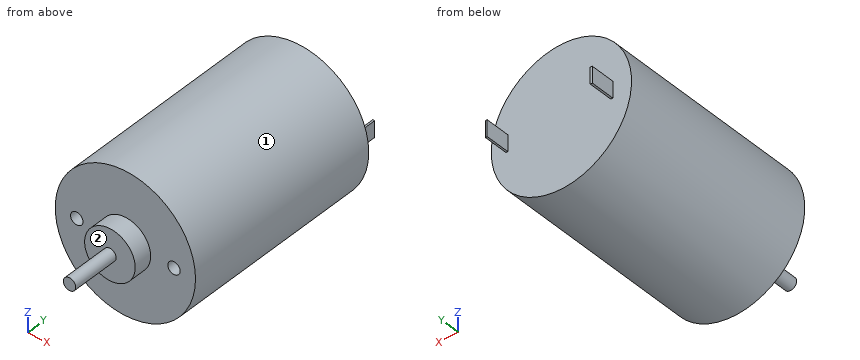
Autodesk Inventor part; units mm, degrees
ref_plane "YZ Plane" through (0, 0, 0) normal (1, 0, 0) x (0, 1, 0)
ref_plane "XZ Plane" through (0, 0, 0) normal (0, 1, 0) x (-1, 0, 0)
ref_plane "XY Plane" through (0, 0, 0) normal (0, 0, 1) x (1, 0, 0)
sketch "Sketch1" plane through (0, 0, 0) normal (0, 0, 1) x (1, 0, 0)
  line L0 (0, 0) -> (1.6, 0)
  line L1 (1.6, 0) -> (1.6, 12.446)
  line L2 (0, 17.2085) -> (18.034, 17.2085)
  line L3 (0, 12.446) -> (6.5, 12.446)
  line L4 (6.5, 12.446) -> (6.5, 17.2085)
  line L5 (18.034, 17.2085) -> (18.034, 70.5485)
  line L6 (18.034, 70.5485) -> (0, 70.5485)
  line L7 (0, 70.5485) -> (0, 0)
  dimension "d0" = 1.6
  dimension "d1" = 12.446
  dimension "d2" = 18.034
  dimension "d3" = 6.5
  dimension "d4" = 4.7625
  dimension "d5" = 53.34
revolve "Revolution1" add sketch "Sketch1" angle 360 about axis through (0, 70.5485, 0) along (0, -1, 0)
sketch "Sketch2" plane through (0, 17.2085, 0) normal (0, -1, 0) x (1, 0, 0)
  circle A0 centre (0, 0) radius 12.5
  circle A1 centre (-12.5, 0) radius 1.6
  circle A2 centre (12.5, 0) radius 1.6
  point P0 (0, 0)
  dimension "d7" = 25
  dimension "d8" = 3.2
  dimension "d9" = 3.2
extrude "Extrusion1" cut sketch "Sketch2" against normal blind 6.35 contours A0 A2 | A0 A2 | A1 A0 | A0 A1
sketch "Sketch3" plane through (0, 70.5485, 0) normal (0, 1, 0) x (1, 0, 0)
  line L0 (14.2427, 1.9025) -> (13.7699, 1.9025)
  line L1 (13.7699, 1.9025) -> (13.7699, -2.2939)
  line L2 (13.7699, -2.2939) -> (14.2427, -2.2939)
  line L3 (14.2427, -2.2939) -> (14.2427, 1.9025)
  line L4 (-12.709, 1.9025) -> (-13.2409, 1.9025)
  line L5 (-13.2409, 1.9025) -> (-13.2409, -2.2939)
  line L6 (-13.2409, -2.2939) -> (-12.709, -2.2939)
  line L7 (-12.709, -2.2939) -> (-12.709, 1.9025)
  point P0 (0, 0)
extrude "Extrusion2" add sketch "Sketch3" along normal blind 6.35
properties part number "540DCMotor"
For this review, take the finished solid that the model builds, in its own axes (mm). Face numbers are marked on the shaded views. A direction names the side the tool comes from. Round coordinates to 2 decimals unless told otherwise and drop trailing zeros. Write each loop counter-clockwise with the first axis right and the second up, starting at its lowest first coordinate (ties: lowest second). Pieces come first, ordered by that corner, then holes. Notation, with made-up numbers: (31.25, -38) -> (71.25, -38) arc R10 ccw to (71.25, -19) -> close; hole circle Ø11 at (7.25, 8). An arc over 180 degrees is marked (long way). One line per question, with ' | ' between items. Start each with the question number.
(1) Add section D-D, the plane x = 12.5. Write out the cut boundary in (y, z), plus the area to 3 significant figures.
(2) For line 1 along X through (y, z) = (72, 1.5); line 2 along Y through (x, z) = (-5.5, -8); line 3 along Z through (x, y) = (12.5, 19.5), list the stretches that pass through material, from the lowest coordinate up. Write a range as from..to.
(3) Add section C-C, the plane y = 57.5. Write out the cut boundary in (x, z), plus the area to 3 significant figures.
(4) Add section A-A, the plane x = 0. Write out the cut boundary in (y, z), plus the area to 3 significant figures.
(5) Insertion check: P1, Ø3.5, axis at y = 72.5, z = 1, coming from the +X side; P2, Ø2, axis at x = 2.5, y = 20, coming from the -Z side; P3, Ø2, axis at x = 7, z = -7.5, coming from the -Y side. Each pin has a flat end and moves straight along its axis. Give the tip position at first contact, or say it passes through.
(6) Add section B-B, the plane z = 0. Write out the cut boundary in (x, y), plus the area to 3 significant figures.
(7) Tool access review of the marked faces 1 and 2: name each direction out of +Z, -Z, +X, -X, +Y, -Y from which nothing blocks a thin tool from reaching the whole face with its end or side.
Answer list:
1) outline: (17.21, -13) -> (70.55, -13) -> (70.55, 13) -> (17.21, 13) -> (17.21, 1.6) -> (23.56, 1.6) -> (23.56, -1.6) -> (17.21, -1.6) -> close | area: 1,370 mm²
2) line 1: -13.24..-12.71, 13.77..14.24 | line 2: 17.21..70.55 | line 3: -13..-1.6, 1.6..13
3) outline: circle Ø36.07 at (0, 0) | area: 1,020 mm²
4) outline: (0, -1.6) -> (12.45, -1.6) -> (12.45, -6.5) -> (17.21, -6.5) -> (17.21, -18.03) -> (70.55, -18.03) -> (70.55, 18.03) -> (17.21, 18.03) -> (17.21, 6.5) -> (12.45, 6.5) -> (12.45, 1.6) -> (0, 1.6) -> close | area: 2,030 mm²
5) P1: x = 14.24 | P2: z = -17.97 | P3: y = 17.21
6) outline: (-18.03, 17.21) -> (-14.1, 17.21) -> (-14.1, 23.56) -> (-10.9, 23.56) -> (-10.9, 17.21) -> (-6.5, 17.21) -> (-6.5, 12.45) -> (-1.6, 12.45) -> (-1.6, 0) -> (1.6, 0) -> (1.6, 12.45) -> (6.5, 12.45) -> (6.5, 17.21) -> (10.9, 17.21) -> (10.9, 23.56) -> (14.1, 23.56) -> (14.1, 17.21) -> (18.03, 17.21) -> (18.03, 70.55) -> (14.24, 70.55) -> (14.24, 76.9) -> (13.77, 76.9) -> (13.77, 70.55) -> (-12.71, 70.55) -> (-12.71, 76.9) -> (-13.24, 76.9) -> (-13.24, 70.55) -> (-18.03, 70.55) -> close | area: 1,990 mm²
7) face 1: +Y, -Y | face 2: -Y
